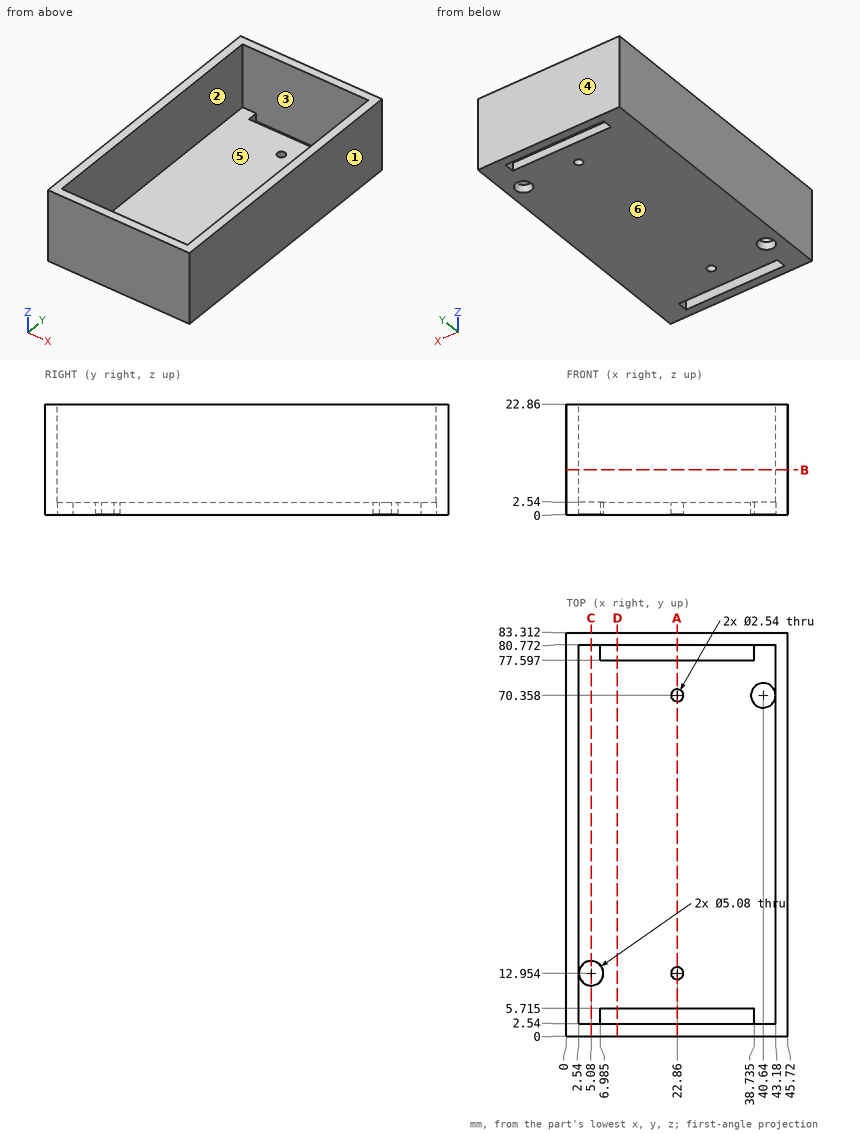
Source: three-view drawing plus pictorial views. Frame: mm from the lowest corner of the part. A direction names the side the tool comes from. Round coordinates to 2 decimals unless told otherwise and drop trailing zeros. Loops run counter-clockwise (first coordinate to the right, second up) from the corner with the lowest first, then second, coordinate; pieces in that order, holes last.
Q1. First-contact query: P1, Ø4, axis at x = 40.64, y = 70.358, coming from the +Z side; P2, Ø20.5, axis at x = 18.5, y = 56.5, coming from the +Z side. Flat tips, straight axial feed; report the tip coordinate or a pass-through.
Q2. Section B-B, the plane z = 9.25. Return loops of the section in (x, y), plus the area to 3 significant figures.
Q3. Access query for the marked faces 1 and 2. Directions: +Z, -Z, +X, -X, +Y, -Y. A direction counts if a zero-diameter tool reaches every point of the face in a straight line with its end or side. Return the directions, or none.
Q4. Section A-A, the plane x = 22.86. Return loops of the section in (y, z) (3 decimals).
Q5. Section C-C, the plane x = 5.08. Return loops of the section in (y, z), plus the area to 3 significant figures.
Q6. Mould query, pull axis Y, two halves, no side actions, for the marked faces 3, 4, 5 and 6. Classes: pulls with the +Y half, pulls with the -Y half, needs draft (parallel to the pull), parting line crosses it, or undercut.
Q7. Section D-D, the plane x = 10.5. Return loops of the section in (y, z) (3 decimals).
Q8. Ray query, line 1 (Y direction, x = 22.86, z = 1.6) (3 decimals); line 2 (Y direction, x = 40.64, z = 0.65); line 3 (X direction, y = 5.5, z = 12.75). Return the intervals inside material, ascending.
Solutions:
1. P1: passes through
1. P2: stops at z = 2.54
2. outline: (0, 0) - (45.72, 0) - (45.72, 83.31) - (0, 83.31) - close; hole (2.54, 2.54) - (43.18, 2.54) - (43.18, 80.77) - (2.54, 80.77) - close
2. area: 630 mm2
3. face 1: +Z, -Z, +X, +Y, -Y
3. face 2: +Z
4. outline: (0, 0) - (2.54, 0) - (2.54, 22.86) - (0, 22.86) - close; (5.715, 0) - (11.684, 0) - (11.684, 2.54) - (5.715, 2.54) - close; (14.224, 0) - (69.088, 0) - (69.088, 2.54) - (14.224, 2.54) - close; (71.628, 0) - (77.597, 0) - (77.597, 2.54) - (71.628, 2.54) - close; (80.772, 0) - (83.312, 0) - (83.312, 22.86) - (80.772, 22.86) - close
5. outline: (0, 0) - (10.41, 0) - (10.41, 2.54) - (2.54, 2.54) - (2.54, 22.86) - (0, 22.86) - close; (15.49, 0) - (83.31, 0) - (83.31, 22.86) - (80.77, 22.86) - (80.77, 2.54) - (15.49, 2.54) - close
5. area: 302 mm2
6. face 3: undercut
6. face 4: pulls with the +Y half
6. face 5: undercut
6. face 6: needs draft
7. outline: (0, 0) - (2.54, 0) - (2.54, 22.86) - (0, 22.86) - close; (5.715, 0) - (77.597, 0) - (77.597, 2.54) - (5.715, 2.54) - close; (80.772, 0) - (83.312, 0) - (83.312, 22.86) - (80.772, 22.86) - close
8. line 1: y = 0 to 2.54, 5.715 to 11.684, 14.224 to 69.088, 71.628 to 77.597, 80.772 to 83.312
8. line 2: y = 0 to 67.82, 72.9 to 83.31
8. line 3: x = 0 to 2.54, 43.18 to 45.72
